from build123d import *

# Parameters (mm, degrees)
SKETCH2_W           = 15
SKETCH2_H           = 19
BOSS_EXTRUDE1_DEPTH = 10
SKETCH3_W           = 15
SKETCH3_H           = 19
BOSS_EXTRUDE2_DEPTH = 2
FILLET1_R           = 1.5
FILLET3_R           = 1.5


with BuildPart() as part:
    # Sketch2 → Boss-Extrude1 (new body)
    with BuildSketch(Plane(origin=(0, 0, 0), x_dir=(1, 0, 0), z_dir=(0, 1, 0))):
        with Locations((7.5, 9.5)):
            Rectangle(SKETCH2_W, SKETCH2_H)
    extrude(amount=BOSS_EXTRUDE1_DEPTH)

    # Sketch3 → Boss-Extrude2 (add)
    with BuildSketch(Plane(origin=(0, 10, 0), x_dir=(1, 0, 0), z_dir=(0, 1, 0))):
        with Locations((7.5, 9.5)):
            Rectangle(SKETCH3_W, SKETCH3_H)
    extrude(amount=BOSS_EXTRUDE2_DEPTH)

    # Fillet1
    fillet1_edges = [part.edges().sort_by_distance(p)[0] for p in [
        (0, 12, -9.5),
        (7.5, 12, 0),
        (15, 12, -9.5),
        (7.5, 12, -19),
    ]]
    fillet(fillet1_edges, radius=FILLET1_R)

    # Fillet3
    # the kernel refuses this fillet: 1.5 mm, written as the material it takes off along each edge
    with BuildSketch(Plane(origin=(13.5, 10.5, -1.5), x_dir=(1, 0, 0), z_dir=(0, 0, 1))) as fillet3_piece_1_section:
        Polygon((0, 0), (FILLET3_R, 0), (FILLET3_R, FILLET3_R), (0, FILLET3_R), align=None)
    fillet3_piece_1 = extrude(amount=FILLET3_R, mode=Mode.PRIVATE)
    fillet3_piece_1 = fillet3_piece_1 - Plane(origin=(13.5, 10.5, -1.5), x_dir=(-0.7071067811865475, -0.7071067811865475, 0), z_dir=(0, 0, 1)) * Sphere(FILLET3_R, mode=Mode.PRIVATE)
    add(fillet3_piece_1, mode=Mode.SUBTRACT)
    with BuildSketch(Plane(origin=(1.5, 10.5, -1.5), x_dir=(-1, 0, 0), z_dir=(0, 0, 1))) as fillet3_piece_2_section:
        Polygon((0, 0), (FILLET3_R, 0), (FILLET3_R, -FILLET3_R), (0, -FILLET3_R), align=None)
    fillet3_piece_2 = extrude(amount=FILLET3_R, mode=Mode.PRIVATE)
    fillet3_piece_2 = fillet3_piece_2 - Plane(origin=(1.5, 10.5, -1.5), x_dir=(0.7071067811865475, -0.7071067811865475, 0), z_dir=(0, 0, 1)) * Sphere(FILLET3_R, mode=Mode.PRIVATE)
    add(fillet3_piece_2, mode=Mode.SUBTRACT)
    with BuildSketch(Plane(origin=(13.5, 10.5, -17.5), x_dir=(0, 0, -1), z_dir=(1, 0, 0))) as fillet3_piece_3_section:
        Polygon((0, 0), (FILLET3_R, 0), (FILLET3_R, FILLET3_R), (0, FILLET3_R), align=None)
    fillet3_piece_3 = extrude(amount=FILLET3_R, mode=Mode.PRIVATE)
    fillet3_piece_3 = fillet3_piece_3 - Plane(origin=(13.5, 10.5, -17.5), x_dir=(0, -0.7071067811865475, 0.7071067811865475), z_dir=(1, 0, 0)) * Sphere(FILLET3_R, mode=Mode.PRIVATE)
    add(fillet3_piece_3, mode=Mode.SUBTRACT)
    with BuildSketch(Plane(origin=(1.5, 10.5, -17.5), x_dir=(0, 0, -1), z_dir=(-1, 0, 0))) as fillet3_piece_4_section:
        Polygon((0, 0), (FILLET3_R, 0), (FILLET3_R, -FILLET3_R), (0, -FILLET3_R), align=None)
    fillet3_piece_4 = extrude(amount=FILLET3_R, mode=Mode.PRIVATE)
    fillet3_piece_4 = fillet3_piece_4 - Plane(origin=(1.5, 10.5, -17.5), x_dir=(0, -0.7071067811865475, 0.7071067811865475), z_dir=(-1, 0, 0)) * Sphere(FILLET3_R, mode=Mode.PRIVATE)
    add(fillet3_piece_4, mode=Mode.SUBTRACT)
    with BuildSketch(Plane(origin=(0, 10.5, -19), x_dir=(0, 0, 1), z_dir=(0, -1, 0)), Plane(origin=(15, -3.75, -19), x_dir=(0, 0, 1), z_dir=(0, 1, 0)), Plane(origin=(15, -3.75, 0), x_dir=(-1, 0, 0), z_dir=(0, 1, 0)), Plane(origin=(0, 10.5, 0), x_dir=(1, 0, 0), z_dir=(0, -1, 0))) as fillet3_piece_5:
        with BuildLine():
            CenterArc((FILLET3_R, -FILLET3_R), FILLET3_R, 90, 90)
            Line((0, -FILLET3_R), (0, 0))
            Line((0, 0), (FILLET3_R, 0))
        make_face()
    extrude(amount=14.25, mode=Mode.SUBTRACT)


solid = part.part
Verification items for the finished model (mm, model axes). Coordinates: 2 decimals unless noted, no trailing zeros. Order: outer loops, then holes, each group sorted by start corner. A loop starts at its lowest first (then second) coordinate and runs counter-clockwise, first axis right, second up. Notation, with made-up numbers: (17.5, 56.5) -> (36.5, 56.5) arc R12 ccw to (36.5, 77.5) -> close; hole circle Ø11 at (65, 7.25). An arc over 180 degrees is marked (long way). Put each result on its own line as item: value. Start each with the question number.
1. Material ranges on L1, parallel to Z at x = 13.75, y = 6; L2, parallel to Y at x = 14, z = -4.5; L3, parallel to Y at x = 14.5, z = -11.25, recorded low to high. Write a range as [from, to].
2. Cross-section at B-B, the plane x = 1. Record the boundary of the cut face in (y, z), then the cut area to 3 significant figures.
3. Cross-section at A-A, the plane y = 11. Record the boundary of the cut face in (x, z), then the cut area to 3 significant figures.
4. Mould release check, pull along Z, two halves, no side actions. Record for faces 1 (the cylindrical face through (14.55, 5.18, -0.43)), 2 (the cylindrical face through (7.58, 11.55, -18.57)), 3 (the cylindrical face through (14.57, 11.55, -9.61)): released by +Z, released by -Z, zero draft, split by the parting line, or undercut.
Computed:
1. L1: [-18.98, -0.02]
1. L2: [0, 11.91]
1. L3: [0, 11.62]
2. outline: (0, -18.91) -> (10.5, -18.91) arc R1.41 ccw to (11.91, -17.5) -> (11.91, -1.5) arc R1.41 ccw to (10.5, -0.09) -> (0, -0.09) -> close
2. area: 223 mm2
3. outline: (0.09, -17.5) arc R1.41 ccw to (1.5, -18.91) -> (13.5, -18.91) arc R1.41 ccw to (14.91, -17.5) -> (14.91, -1.5) arc R1.41 ccw to (13.5, -0.09) -> (1.5, -0.09) arc R1.41 ccw to (0.09, -1.5) -> close
3. area: 277 mm2
4. face 1: released by +Z
4. face 2: released by -Z
4. face 3: zero draft
